from build123d import *

# Parameters (mm, degrees)
CYLINDER_R     = 3
CYLINDER_DEPTH = 10
BOX_W          = 120
BOX_H          = 120
BOX_DEPTH      = 1.6


with BuildPart() as cylinder:
    # Cylinder → Cylinder (new body)
    with BuildSketch(Plane(origin=(7.5, 30.5, -5), x_dir=(1, 0, 0), z_dir=(0, 0, 1))):
        Circle(CYLINDER_R)
    extrude(amount=CYLINDER_DEPTH)


with BuildPart() as clone_of_cylinder001:
    # Clone001 base: copy of Cylinder
    add(cylinder.part)


with BuildPart() as clone_of_cylinder001_1:
    # Clone001 placement: moved
    add(clone_of_cylinder001.part.moved(Location((105, 0, 0))))


with BuildPart() as clone_of_cylinder:
    # Clone base: copy of Cylinder
    add(cylinder.part)


with BuildPart() as clone_of_cylinder_1:
    # Clone placement: moved
    add(clone_of_cylinder.part.moved(Location((0, 82.5, 0))))


with BuildPart() as clone_of_cylinder002:
    # Clone002 base: copy of Cylinder
    add(cylinder.part)


with BuildPart() as clone_of_cylinder002_1:
    # Clone002 placement: moved
    add(clone_of_cylinder002.part.moved(Location((105, 82.5, 0))))


with BuildPart() as fusion:
    # Fusion base: copy of Cylinder
    add(cylinder.part)

    # Fusion: union Clone of Cylinder001, Clone of Cylinder, Clone of Cylinder002
    add(clone_of_cylinder001_1.part)
    add(clone_of_cylinder_1.part)
    add(clone_of_cylinder002_1.part)


with BuildPart() as board:
    # Box → Box (new body)
    with BuildSketch(Plane.XY):
        with Locations((60, 60)):
            Rectangle(BOX_W, BOX_H)
    extrude(amount=BOX_DEPTH)

    # Cut: cut Fusion
    add(fusion.part, mode=Mode.SUBTRACT)


solid = board.part
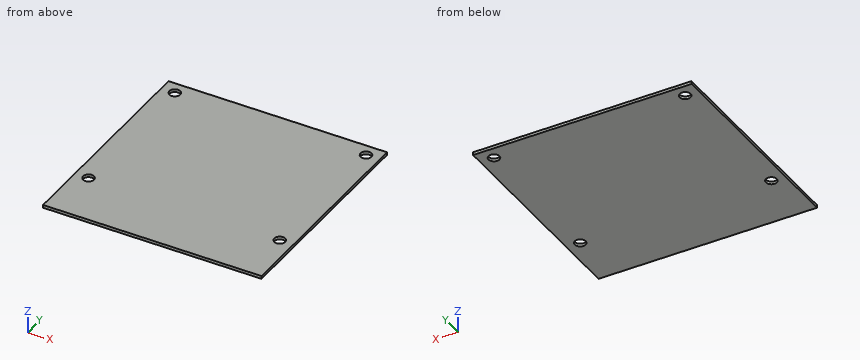
The model under review builds one solid part; all positions refer to its coordinate system, in mm. Round coordinates to 2 decimals unless told otherwise and drop trailing zeros. Order: outer loops, then holes, each group sorted by start corner. A loop starts at its lowest first (then second) coordinate and runs counter-clockwise, first axis right, second up. Notation, with made-up numbers: (88, 56) -> (117, 56) arc R25 cw to (117, 74) -> close; hole circle Ø8 at (-26, 59). An arc over 180 degrees is marked (long way). Use CSV: the item, a comma, the result in double quotes. Start each with the question number.
(1) Consider section B-B on y = 30.5. Write out the cut boundary in (x, z), and give its area (3 significant figures).
(2) Wall thickness on probe 1 along Y at (x, z) = (112.5, 1); probe 2 along X at (y, z) = (30.5, 0.85): over which ranges is each line inside the solid? List them lowest first. Write a range as from..to.
(3) Consider section A-A on x = 7.5. Write out the cut boundary in (y, z).
Responses:
1,outline,"(0, 0) -> (4.5, 0) -> (4.5, 1.6) -> (0, 1.6) -> close; (10.5, 0) -> (109.5, 0) -> (109.5, 1.6) -> (10.5, 1.6) -> close; (115.5, 0) -> (120, 0) -> (120, 1.6) -> (115.5, 1.6) -> close"
1,area,"173 mm²"
2,probe 1,"0..27.5, 33.5..110, 116..120"
2,probe 2,"0..4.5, 10.5..109.5, 115.5..120"
3,outline,"(0, 0) -> (27.5, 0) -> (27.5, 1.6) -> (0, 1.6) -> close; (33.5, 0) -> (110, 0) -> (110, 1.6) -> (33.5, 1.6) -> close; (116, 0) -> (120, 0) -> (120, 1.6) -> (116, 1.6) -> close"
